```python
from build123d import *

# Parameters (mm, degrees)
SKETCH1_R           = 2
SKETCH1_R_2         = 1
BOSS_EXTRUDE1_DEPTH = 1.2
FILLET1_R           = 1


with BuildPart() as part:
    # Sketch1 → Boss-Extrude1 (new body)
    with BuildSketch(Plane(origin=(0, 0, 0), x_dir=(1, 0, 0), z_dir=(0, 1, 0))):
        with BuildLine():
            ThreePointArc((-19.691368668, 3.5), (-23.513581264, 0), (-19.691368668, -3.5))
            Line((-19.691368668, -3.5), (-9.367496998, -3.5))
            ThreePointArc((-9.367496998, -3.5), (-7.660444431, -6.427876097), (-5.073475918, -8.617415048))
            Line((-5.073475918, -8.617415048), (-6.86619742, -18.784443909))
            ThreePointArc((-6.86619742, -18.784443909), (-4.083090537, -23.15635713), (0.027456851, -19.999981153))
            Line((0.027456851, -19.999981153), (1.776996571, -10.077848346))
            Line((1.776996571, -10.077848346), (6.814595421, -18.803225501))
            ThreePointArc((6.814595421, -18.803225501), (11.756790632, -20.363358709), (12.876773247, -15.303225501))
            Line((12.876773247, -15.303225501), (7.714837412, -6.36249037))
            ThreePointArc((7.714837412, -6.36249037), (9.396926208, -3.420201433), (9.999638306, -0.085051507))
            Line((9.999638306, -0.085051507), (19.700904332, 3.445920561))
            ThreePointArc((19.700904332, 3.445920561), (22.095538802, 8.042118434), (17.306763328, 10.023768907))
            Line((17.306763328, 10.023768907), (7.839174397, 6.577848346))
            Line((7.839174397, 6.577848346), (12.876773247, 15.303225501))
            ThreePointArc((12.876773247, 15.303225501), (11.756790632, 20.363358709), (6.814595421, 18.803225501))
            Line((6.814595421, 18.803225501), (1.652659586, 9.86249037))
            ThreePointArc((1.652659586, 9.86249037), (-1.736481777, 9.84807753), (-4.926162387, 8.702466555))
            Line((-4.926162387, 8.702466555), (-12.834706911, 15.338523348))
            ThreePointArc((-12.834706911, 15.338523348), (-18.012448265, 15.114238696), (-17.334220179, 9.976212246))
            Line((-17.334220179, 9.976212246), (-9.616170968, 3.5))
            Line((-9.616170968, 3.5), (-19.691368668, 3.5))
        make_face()
        with Locations((-20, 0)):
            Circle(SKETCH1_R, mode=Mode.SUBTRACT)
        Polygon((-14, -1), (-14, 0), (-13, 0), align=None, mode=Mode.SUBTRACT)
        with Locations((5.745333323, 4.820907073)):
            Circle(SKETCH1_R_2, mode=Mode.SUBTRACT)
        with Locations((1.302361333, -7.386058148)):
            Circle(SKETCH1_R_2, mode=Mode.SUBTRACT)
        with Locations((-7.047694656, 2.565151075)):
            Circle(SKETCH1_R_2, mode=Mode.SUBTRACT)
        Polygon((-2.25742631, -12.802500789), (-1.446266734, -13.96095672), (-2.431074487, -13.787308542), align=None, mode=Mode.SUBTRACT)
        with Locations((-3.472963553, -19.69615506)):
            Circle(SKETCH1_R, mode=Mode.SUBTRACT)
        with Locations((-15.320888862, 12.855752194)):
            Circle(SKETCH1_R, mode=Mode.SUBTRACT)
        Polygon((-10.724622204, 8.999026536), (-9.958577761, 8.356238926), (-11.367409813, 8.232982092), align=None, mode=Mode.SUBTRACT)
        Polygon((7, -12.124355653), (6.5, -11.258330249), (7.866025404, -11.624355653), align=None, mode=Mode.SUBTRACT)
        with Locations((10, -17.320508076)):
            Circle(SKETCH1_R, mode=Mode.SUBTRACT)
        with Locations((10, 17.320508076)):
            Circle(SKETCH1_R, mode=Mode.SUBTRACT)
        Polygon((6.133974596, 12.624355653), (7, 12.124355653), (6.5, 11.258330249), align=None, mode=Mode.SUBTRACT)
        with Locations((18.793852416, 6.840402867)):
            Circle(SKETCH1_R, mode=Mode.SUBTRACT)
        Polygon((13.155696691, 4.788282007), (12.21600407, 4.446261863), (12.813676548, 5.727974627), align=None, mode=Mode.SUBTRACT)
    extrude(amount=BOSS_EXTRUDE1_DEPTH)

    # Fillet1
    fillet1_edges = [part.edges().sort_by_distance(p)[0] for p in [
        (17.306763328, 0.6, -10.023768907),
        (19.700904332, 0.6, -3.445920561),
        (9.999638306, 0.6, 0.085051507),
        (7.714837412, 0.6, 6.36249037),
        (12.876773247, 0.6, 15.303225501),
        (6.814595421, 0.6, 18.803225501),
        (1.776996571, 0.6, 10.077848346),
        (0.027456851, 0.6, 19.999981153),
        (-6.86619742, 0.6, 18.784443909),
        (-5.073475918, 0.6, 8.617415048),
        (-9.367496998, 0.6, 3.5),
        (-19.691368668, 0.6, 3.5),
        (-19.691368668, 0.6, -3.5),
        (-9.616170968, 0.6, -3.5),
        (-17.334220179, 0.6, -9.976212246),
        (-12.834706911, 0.6, -15.338523348),
        (-4.926162387, 0.6, -8.702466555),
        (1.652659586, 0.6, -9.86249037),
        (6.814595421, 0.6, -18.803225501),
        (12.876773247, 0.6, -15.303225501),
        (7.839174397, 0.6, -6.577848346),
    ]]
    fillet(fillet1_edges, radius=FILLET1_R)


solid = part.part
```
Verification items for the finished model (mm, model axes). A direction names the side the tool comes from. Coordinates: 2 decimals unless noted, no trailing zeros. Order: outer loops, then holes, each group sorted by start corner. A loop starts at its lowest first (then second) coordinate and runs counter-clockwise, first axis right, second up. Notation, with made-up numbers: (-27, 84.25) - (17, 84.25) arc R19 ccw to (17, 106.25) - close; hole circle Ø3 at (13.5, 62). An arc over 180 degrees is marked (long way). Return JSON: item names as keys, results as strings.
(1) Section check A-A, the plane x = 4. Record the cut outline in (y, z), and give its area (3 significant figures).
Filled sheet:
{"outline": "(0, -13.93) - (1.2, -13.93) - (1.2, 13.93) - (0, 13.93) - close", "area": "33.4 mm^2"}
(2) Thickness scan on line 1 along X through (y, z) = (1, 20); line 2 along Z through (x, y) = (-20, 0.35); line 3 along X through (y, z) = (0.6, 17.5). Record the ranges inside material, lowest first.
Filled sheet:
{"line 1": "x = -6.97 to -5.45, -1.5 to 0.03, 7.73 to 12.27", "line 2": "z = -3.51 to -2, 2 to 3.51", "line 3": "x = -6.64 to 0.47, 6.06 to 8.01, 11.99 to 13.51"}
(3) Section check B-B, the plane y = 0.7. Give the number of separate pieces and of enclosed holes in the cut face, and give its area (3 significant figures).
Filled sheet:
{"separate pieces": "1", "enclosed holes": "15", "area": "776 mm^2"}
(4) Access from +Z, -Z, +X, -X, +Y, -Y to the whole of each face (thin tool, end or side, straight path). Record for faces 1 (the flat face through (4.435, 0.592, -14.681)), 2 (the cylindrical face through (9.384, 0.592, 3.457)), 3 (the flat face through (13.912, 0.592, -8.788)).
Filled sheet:
{"face 1": "-Z, +Y, -Y", "face 2": "+X, +Y, -Y", "face 3": "+Y, -Y"}
(5) Mould release check, pull along Z, two halves, no side actions. Record for faces 4 (the cylindrical face through (-3.733, 0.592, 17.713)), 5 (the cylindrical face through (-11.43, 0.61, -4.14)), 6 (the flat face through (-9.085, 0.592, -12.192)): pulls with the +Z half, pulls with the -Z half, needs draft (parallel to the pull), parting line crosses it, or undercut.
Filled sheet:
{"face 4": "undercut", "face 5": "undercut", "face 6": "pulls with the -Z half"}
